Verification items for the finished model (mm, model axes). Face numbers are marked on the shaded views. A direction names the side the tool comes from. Coordinates: 2 decimals unless noted, no trailing zeros. Order: outer loops, then holes, each group sorted by start corner. A loop starts at its lowest first (then second) coordinate and runs counter-clockwise, first axis right, second up. Notation, with made-up numbers: M 7,3 L 56,3 A17 cw 56,13 Z; hole C -4,60.25 d1. An arc over 180 degrees is marked long. Write item = value, one per line.
```python
from build123d import *

# Parameters (mm, degrees)
F1_DEPTH = 6.5
F2_R     = 1.65
F3_DEPTH = 31.001
F4_R     = 0.5
F5_R     = 1


with BuildPart() as f1:
    # F0 (on Top) → F1 (new body)
    with BuildSketch(Plane.XY):
        Polygon((15, 0), (-15, 0), (-15, 19), (-15.5, 19), (-15.5, -0.5), (15.5, -0.5), (15.5, 19), (15, 19), align=None)
    extrude(amount=F1_DEPTH)

    # F2 (on face) → F3 (cut, through all)
    with BuildSketch(Plane.YZ.offset(15.5)):
        with Locations((12, 3.25)):
            Circle(F2_R)
    extrude(amount=-F3_DEPTH, mode=Mode.SUBTRACT)

    # F4
    f4_edges = [f1.edges().sort_by_distance(p)[0] for p in [
        (-15.5, -0.5, 3.25),
        (15.5, -0.5, 3.25),
        (15, 0, 3.25),
        (-15, 0, 3.25),
    ]]
    fillet(f4_edges, radius=F4_R)

    # F5
    f5_edges = [f1.edges().sort_by_distance(p)[0] for p in [
        (-15.25, 19, 6.5),
        (-15.25, 19, 0),
        (15.25, 19, 6.5),
        (15.25, 19, 0),
    ]]
    fillet(f5_edges, radius=F5_R)


solid = f1.part
```
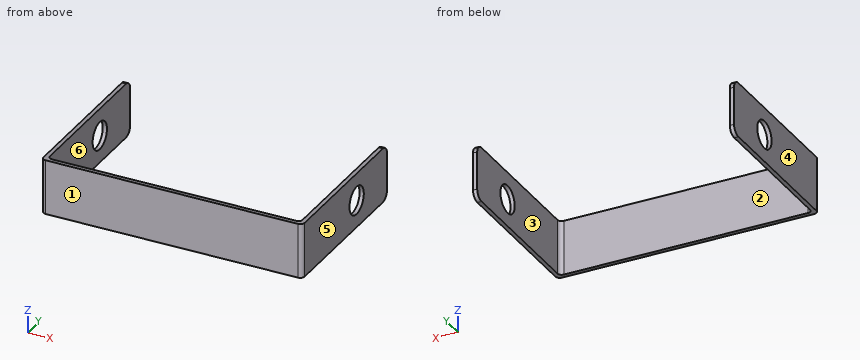
Item 1: Tool access check on the marked faces 1 and 2. Record the directions out of +Z, -Z, +X, -X, +Y, -Y that give a thin tool (end or side, any length) a straight path to the whole face; none if there is none.
Report:
face_1 = +Z, -Z, +X, -X, -Y
face_2 = +Z, -Z, +Y
Item 2: Scan lines: L1, parallel to X at y = 17.25, z = 5.5; L2, parallel to Z at x = 15.2, y = 12; L3, parallel to Y at x = -7, z = 2. Record each from-to range of solid material in increasing order. Write a range as from..to.
Report:
L1 = -15.5..-15, 15..15.5
L2 = 0..1.6, 4.9..6.5
L3 = -0.5..0
Item 3: Gauge pin test, flat end, axial feed: pin 1 (2.5 mm diameter, centred on y = 12, z = 3.25, fed in from -X). Record the tip position at first contact, or that the pin passes through.
Report:
pin_1 = through
Item 4: Release check for a two-part mould opening along X. For the marked faces 3, 4, 5 and 6 record: pulls with the +X half, pulls with the -X half, needs draft (parallel to the pull), parting line crosses it, or undercut.
Report:
face_3 = undercut
face_4 = pulls with the -X half
face_5 = pulls with the +X half
face_6 = undercut
Item 5: Sectioned sample at B-B, the plane z = 3.25. Enter the section's corners in (x, y), then the cut area to 3 significant figures.
Report:
outline = M -15.5,0 A0.5 ccw -15,-0.5 L 15,-0.5 A0.5 ccw 15.5,0 L 15.5,10.35 L 15,10.35 L 15,0.5 A0.5 cw 14.5,0 L -14.5,0 A0.5 cw -15,0.5 L -15,10.35 L -15.5,10.35 Z; M -15.5,13.65 L -15,13.65 L -15,19 L -15.5,19 Z; M 15,13.65 L 15.5,13.65 L 15.5,19 L 15,19 Z
area = 31.2 mm^2
Item 6: Sectioned sample at D-D, the plane x = 9. Enter the section's corners in (y, z).
Report:
outline = M -0.5,0 L 0,0 L 0,6.5 L -0.5,6.5 Z
Item 7: Sectioned sample at A-A, the plane y = 12. Enter the section's corners in (x, z), then the cut area to 3 significant figures.
Report:
outline = M -15.5,0 L -15,0 L -15,1.6 L -15.5,1.6 Z; M -15.5,4.9 L -15,4.9 L -15,6.5 L -15.5,6.5 Z; M 15,0 L 15.5,0 L 15.5,1.6 L 15,1.6 Z; M 15,4.9 L 15.5,4.9 L 15.5,6.5 L 15,6.5 Z
area = 3.20 mm^2
Item 8: Sectioned sample at C-C, the plane y = 14. Enter the section's corners in (x, z), then the cut area to 3 significant figures.
Report:
outline = M -15.5,0 L -15,0 L -15,6.5 L -15.5,6.5 Z; M 15,0 L 15.5,0 L 15.5,6.5 L 15,6.5 Z
area = 6.50 mm^2
